from build123d import *

# Parameters (mm, degrees)
SK_ALA_1_W           = 19.05
SK_ALA_1_H           = 3.175
ALA_1_DEPTH          = 20
SK_ALA_2_W           = 3.175
SK_ALA_2_H           = 19.05
ALA_2_DEPTH          = 20
SK_BARRENOS_ALA_1_R  = 2.25
BARRENOS_ALA_1_DEPTH = 3.175
SK_BARRENOS_ALA_2_R  = 2.25
BARRENOS_ALA_2_DEPTH = 3.175


with BuildPart() as part:
    # Sk_Ala_1 → Ala_1 (new body)
    with BuildSketch(Plane.XY):
        with Locations((9.525, 1.5875)):
            Rectangle(SK_ALA_1_W, SK_ALA_1_H)
    extrude(amount=ALA_1_DEPTH)

    # Sk_Ala_2 → Ala_2 (add)
    with BuildSketch(Plane.XY):
        with Locations((1.5875, 9.525)):
            Rectangle(SK_ALA_2_W, SK_ALA_2_H)
    extrude(amount=ALA_2_DEPTH)

    # Sk_Barrenos_ala_1 → Barrenos_ala_1 (cut)
    with BuildSketch(Plane(origin=(0, 0, 0), x_dir=(1, 0, 0), z_dir=(0, 1, 0))):
        with Locations(Location((11.1125, -6, 0), (0, 0, 270))):
            Circle(SK_BARRENOS_ALA_1_R)
        with Locations(Location((11.1125, -16, 0), (0, 0, 270))):
            Circle(SK_BARRENOS_ALA_1_R)
    extrude(amount=BARRENOS_ALA_1_DEPTH, mode=Mode.SUBTRACT)

    # Sk_Barrenos_ala_2 → Barrenos_ala_2 (cut)
    with BuildSketch(Plane(origin=(0, 0, 0), x_dir=(0, 0, -1), z_dir=(1, 0, 0))):
        with Locations((-6, 11.1125)):
            Circle(SK_BARRENOS_ALA_2_R)
        with Locations((-16, 11.1125)):
            Circle(SK_BARRENOS_ALA_2_R)
    extrude(amount=BARRENOS_ALA_2_DEPTH, mode=Mode.SUBTRACT)


solid = part.part
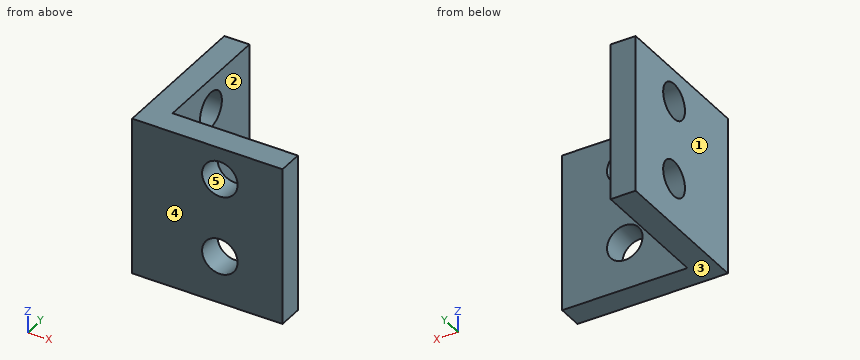
Could you check a few things on this model? Use its own coordinates, in mm. Face numbers are marked on the shaded views. A direction names the side the tool comes from. Give positions to 0.01 mm unless a question says otherwise; leave off trailing zeros. Loops run counter-clockwise (first coordinate to the right, second up) from the corner with the lowest first, then second, coordinate; pieces in that order, holes last. Notation, with made-up numbers: M 67.5,-33.75 L 97.5,-33.75 A30 ccw 97.5,-8.75 Z; hole C 81,50.5 d10. An arc over 180 degrees is marked long. Answer as a JSON object with one key per item and string values.
Q1. Suppose I cut it at C-C, the plane x = 4. List the corners of the cut face in (y, z) for me (3 decimals), plus the area to 3 significant figures.
Values found:
{"outline": "M 0,0 L 3.175,0 L 3.175,20 L 0,20 Z", "area": "63.5 mm²"}
Q2. Suppose I cut it at D-D, the plane z = 10.75. List the corners of the cut face in (x, y) for me (3 decimals), plus the area to 3 significant figures.
Values found:
{"outline": "M 0,0 L 19.05,0 L 19.05,3.175 L 3.175,3.175 L 3.175,19.05 L 0,19.05 Z", "area": "111 mm²"}
Q3. Suppose I cut it at A-A, the plane z = 16. State how many separate pieces and enclosed holes the cut face has, plus the area to 3 significant figures.
Values found:
{"separate pieces": "3", "enclosed holes": "0", "area": "82.3 mm²"}
Q4. Suppose I cut it at B-B, the plane y = 9.75. List the corners of the cut face in (x, z) for me (3 decimals).
Values found:
{"outline": "M 0,0 L 3.175,0 L 3.175,4.209 L 0,4.209 Z; M 0,7.791 L 3.175,7.791 L 3.175,14.209 L 0,14.209 Z; M 0,17.791 L 3.175,17.791 L 3.175,20 L 0,20 Z"}
Q5. For P1, Ø2, axis at x = 9.5, y = 4, coming from the +Z side; P2, Ø4, axis at y = 11.11, z = 6, coming from the +X side; P3, Ø8, axis at y = 13.5, z = 3, coming from the +X side (3 decimals); P4, Ø5, axis at x = 11.11, z = 6, coming from the +Y side (3 decimals), each with a flat end and sliding along its axis, tell me the tip position at first contact or that it passes through.
Values found:
{"P1": "stops at z = 20", "P2": "passes through", "P3": "stops at x = 3.175", "P4": "stops at y = 3.175"}
Q6. If we mould it in two halves opening along Z, with no side actions, what happens to the marked faces 3, 4 and 5? For each: pulls with the +Z half, pulls with the -Z half, needs draft (parallel to the pull), parting line crosses it, or undercut.
Values found:
{"face 3": "pulls with the -Z half", "face 4": "needs draft", "face 5": "undercut"}
Q7. If I drill on probe 1 along X at (y, z) = (2, 16); probe 2 along X at (y, z) = (13.5, 12) (3 decimals), over which ranges is the centre line in solid material (lowest first)? Write a range as [from, to].
Values found:
{"probe 1": "x = [0, 8.86], [13.36, 19.05]", "probe 2": "x = [0, 3.175]"}
Q8. For the marked faces 1 and 2, which set-ups out of +Z, -Z, +X, -X, +Y, -Y let a thin tool reach every point of the face, with its end or its side?
Values found:
{"face 1": "+Z, -Z, -X, +Y, -Y", "face 2": "+Z, -Z, +X, +Y"}
